Answer from the drawing. Dimensions are ordinates in mm from the lowest x, y and z of the part. Coordinates: 2 decimals unless noted, no trailing zeros. Loops run counter-clockwise (first coordinate to the right, second up) from the corner with the lowest first, then second, coordinate; pieces in that order, holes last. Notation, with made-up numbers: (72, 63.25) -> (97, 63.25) arc R9 cw to (97, 70.25) -> close; hole circle Ø10 at (72, 69). An arc over 180 degrees is marked (long way). Use a Markdown table: item, result.
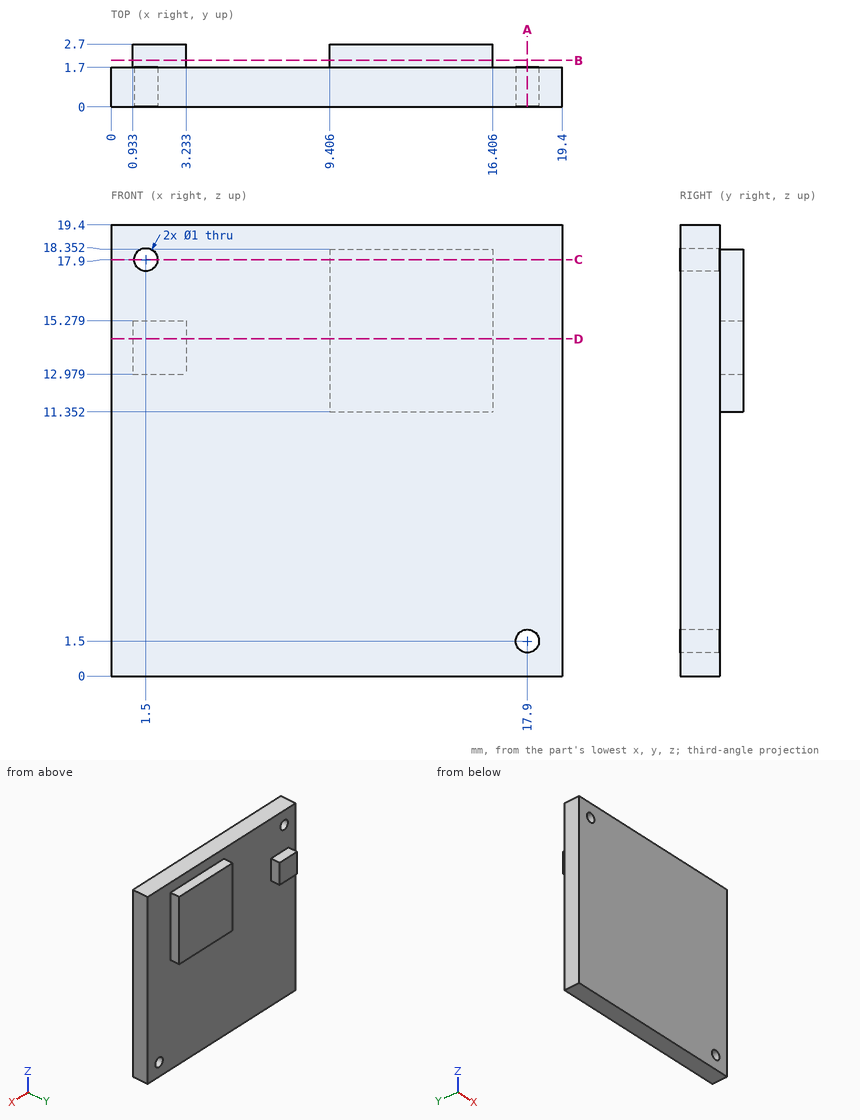
Q1. Section A-A on x = 17.9 is taken. Determine the outline of the cut face in (y, z), and give its area (3 significant figures).
Solved:
| item | result |
|---|---|
| outline | (0, 0) -> (1.7, 0) -> (1.7, 1) -> (0, 1) -> close; (0, 2) -> (1.7, 2) -> (1.7, 19.4) -> (0, 19.4) -> close |
| area | 31.3 mm² |
Q2. Section D-D on z = 14.5 is taken. Determine the outline of the cut face in (x, y), and give its area (3 significant figures).
Solved:
| item | result |
|---|---|
| outline | (0, 0) -> (19.4, 0) -> (19.4, 1.7) -> (16.41, 1.7) -> (16.41, 2.7) -> (9.41, 2.7) -> (9.41, 1.7) -> (3.23, 1.7) -> (3.23, 2.7) -> (0.93, 2.7) -> (0.93, 1.7) -> (0, 1.7) -> close |
| area | 42.3 mm² |
Q3. Section B-B on y = 2 is taken. Determine the outline of the cut face in (x, z), and give its area (3 significant figures).
Solved:
| item | result |
|---|---|
| outline | (0.93, 12.98) -> (3.23, 12.98) -> (3.23, 15.28) -> (0.93, 15.28) -> close; (9.41, 11.35) -> (16.41, 11.35) -> (16.41, 18.35) -> (9.41, 18.35) -> close |
| area | 54.3 mm² |
Q4. Section C-C on z = 17.9 is taken. Determine the outline of the cut face in (x, y).
Solved:
| item | result |
|---|---|
| outline | (0, 0) -> (1, 0) -> (1, 1.7) -> (0, 1.7) -> close; (2, 0) -> (19.4, 0) -> (19.4, 1.7) -> (16.41, 1.7) -> (16.41, 2.7) -> (9.41, 2.7) -> (9.41, 1.7) -> (2, 1.7) -> close |
Q5. Given pin 1 Ø0.5 at (x, y) = (2, 2) entering from -Z; pin 2 Ø0.5 at (y, z) = (2.5, 14.5) entering from -X; pin 3 Ø0.5 at (y, z) = (2, 14) entering from +X, each flat-ended and moving along its own axis, determine where each tip first touches the part or whether it passes through.
Solved:
| item | result |
|---|---|
| pin 1 | z = 12.98 |
| pin 2 | x = 0.93 |
| pin 3 | x = 16.41 |
Q6. Consider line 1 (X direction, y = 0.4, z = 1.5); line 2 (Z direction, x = 17.9, y = 1.3); line 3 (Y direction, x = 8.25, z = 9.5). Determine where each line is inside the solid, lowest interval first. Write a range as [from, to].
Solved:
| item | result |
|---|---|
| line 1 | [0, 17.4], [18.4, 19.4] |
| line 2 | [0, 1], [2, 19.4] |
| line 3 | [0, 1.7] |
